Work out the finished part from the listing and answer in its coordinate system (mm). Round coordinates to 2 decimals unless told otherwise and drop trailing zeros. Write each loop counter-clockwise with the first axis right and the second up, starting at its lowest first coordinate (ties: lowest second). Pieces come first, ordered by that corner, then holes.
from build123d import *

# Parameters (mm, degrees)
SKETCH_1_R          = 2
EXTRUDE_1_DEPTH     = 37.5
CUT_EXTRUDE_START   = -2
SKETCH_2_R          = 2
SKETCH_2_R_2        = 1.5
CUT_EXTRUDE_1_DEPTH = 0.7
CUT_EXTRUDE_START_2 = -1.3
SKETCH_3_R          = 2
SKETCH_3_R_2        = 1.5
CUT_EXTRUDE_2_DEPTH = 0.7


with BuildPart() as part:
    # 스케치1 → 보스-돌출1 (new body)
    with BuildSketch(Plane(origin=(0, 0, 0), x_dir=(1, 0, 0), z_dir=(0, 1, 0))):
        with Locations(Location((0, 0, 0), (0, 0, 270))):
            Circle(SKETCH_1_R)
    extrude(amount=EXTRUDE_1_DEPTH)

    # 스케치2 → 컷-돌출1 (cut)
    with BuildSketch(Plane(origin=(0, 37.5, 0), x_dir=(1, 0, 0), z_dir=(0, 1, 0)).offset(CUT_EXTRUDE_START)):
        with Locations(Location((0, 0, 0), (0, 0, 270))):
            Circle(SKETCH_2_R)
        with Locations(Location((0, 0, 0), (0, 0, 270))):
            Circle(SKETCH_2_R_2, mode=Mode.SUBTRACT)
    extrude(amount=CUT_EXTRUDE_1_DEPTH, mode=Mode.SUBTRACT)

    # 스케치3 → 컷-돌출2 (cut)
    with BuildSketch(Plane.XZ.offset(CUT_EXTRUDE_START_2)):
        with Locations(Location((0, 0, 0), (0, 0, 270))):
            Circle(SKETCH_3_R)
        with Locations(Location((0, 0, 0), (0, 0, 90))):
            Circle(SKETCH_3_R_2, mode=Mode.SUBTRACT)
    extrude(amount=-CUT_EXTRUDE_2_DEPTH, mode=Mode.SUBTRACT)


solid = part.part
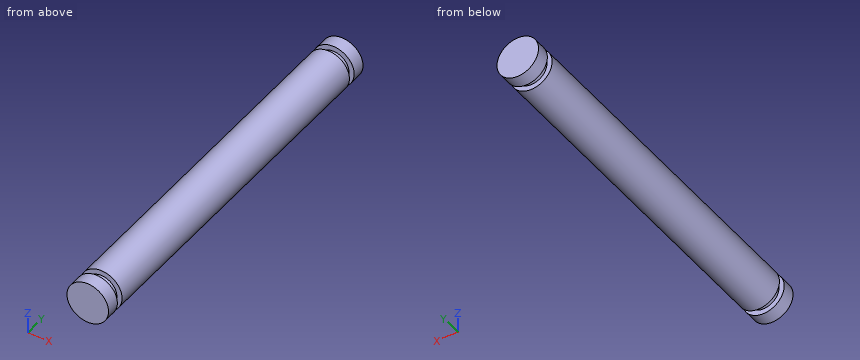
Q1. Find the intervals of material crossed by L1, parallel to Y at x = -1.5, z = -0.9; L2, parallel to X at y = 21, z = 0.1; L3, parallel to Z at x = -0.65, y = 12, in increasing order.
Q2. Find section C-C (z = -0.75). Determine the outline of the cut face in (x, y), plus the area to 4 significant figures.
Q3. Find section A-A (z = 1.05). Determine the outline of the cut face in (x, y), plus the area to 3 significant figures.
Q4. Find section B-B (y = 34.5). Determine the outline of the cut face in (x, z), plus the area to 3 significant figures.
Q5. Given pin 1 (1 mm diameter, centred on y = 23, z = 1.5, fed in from +X); pin 2 (1.2 mm diameter, centred on x = 0.5, z = -0.5, fed in from -Y), each flat-ended and moving along its own axis, determine where each tip first touches the part or whether it passes through.
Report:
1. L1: y = 0 to 1.3, 2 to 35.5, 36.2 to 37.5
1. L2: x = -2 to 2
1. L3: z = -1.89 to 1.89
2. outline: (-1.85, 0) - (1.85, 0) - (1.85, 1.3) - (1.3, 1.3) - (1.3, 2) - (1.85, 2) - (1.85, 35.5) - (1.3, 35.5) - (1.3, 36.2) - (1.85, 36.2) - (1.85, 37.5) - (-1.85, 37.5) - (-1.85, 36.2) - (-1.3, 36.2) - (-1.3, 35.5) - (-1.85, 35.5) - (-1.85, 2) - (-1.3, 2) - (-1.3, 1.3) - (-1.85, 1.3) - close
2. area: 137.5 mm2
3. outline: (-1.7, 0) - (1.7, 0) - (1.7, 1.3) - (1.07, 1.3) - (1.07, 2) - (1.7, 2) - (1.7, 35.5) - (1.07, 35.5) - (1.07, 36.2) - (1.7, 36.2) - (1.7, 37.5) - (-1.7, 37.5) - (-1.7, 36.2) - (-1.07, 36.2) - (-1.07, 35.5) - (-1.7, 35.5) - (-1.7, 2) - (-1.07, 2) - (-1.07, 1.3) - (-1.7, 1.3) - close
3. area: 126 mm2
4. outline: circle Ø4 at (0, 0)
4. area: 12.6 mm2
5. pin 1: stops at x = 1.73
5. pin 2: stops at y = 0
